Read the model definition and answer for the solid it produces. Units are mm, in the model's axes. Give positions to 0.01 mm unless a question says otherwise; leave off trailing zeros. Order: outer loops, then holes, each group sorted by start corner. A loop starts at its lowest first (then second) coordinate and runs counter-clockwise, first axis right, second up. Notation, with made-up numbers: M -35,89.5 L -13,89.5 A20 cw -13,106.5 Z; hole C 49.5,66 d8. An arc over 180 degrees is marked long. One line per item, written item: value.
from build123d import *

# Parameters (mm, degrees)
SM_START                 = -3
SM_BASE_FLANGE_1_DEPTH   = 6
CUT_EXTRUDE_1_DEPTH      = 231.181450165
CUT_EXTRUDE_1_DEPTH_BACK = 231.181450165
SKETCH_7_W               = 4
SKETCH_7_H               = 47
CHAMFER_2_SIZE           = 8
CHAMFER_2_SIZE_2         = 10.078576046
FILLET_1_R               = 6
CHAMFER_3_SIZE           = 4


with BuildPart() as part:
    # Базовая кромка1: read off the stored shape, not the designer's step
    # Базовая кромка1 outline → Базовая кромка1 (new body)
    with BuildSketch(Plane(origin=(0, 0, 0), x_dir=(0, 0, -1), z_dir=(1, 0, 0)).offset(SM_START)):
        with BuildLine():
            Line((-111.5, 0), (-111.5, 146))
            Line((-111.5, 146), (-153.5, 146))
            Line((-153.5, 146), (-153.5, -71.5))
            ThreePointArc((-153.5, -71.5), (-124.210678119, -142.210678119), (-53.5, -171.5))
            Line((-53.5, -171.5), (53.5, -171.5))
            ThreePointArc((53.5, -171.5), (124.210678119, -142.210678119), (153.5, -71.5))
            Line((153.5, -71.5), (153.5, 146))
            Line((153.5, 146), (111.5, 146))
            Line((111.5, 146), (111.5, 0))
            ThreePointArc((111.5, 0), (0, -111.5), (-111.5, 0))
        make_face()
    extrude(amount=SM_BASE_FLANGE_1_DEPTH)

    # Эскиз7 → Вырез-Вытянуть1 (cut, two sides: drawn at the far end of the back side and taken through both)
    with BuildSketch(Plane(origin=(0, 0, 0), x_dir=(0, 0, -1), z_dir=(1, 0, 0)).offset(-CUT_EXTRUDE_1_DEPTH_BACK)):
        Polygon((72.938816537, -84.333736086), (36.565749578, -105.333736086), (57.565749578, -141.706803045), (93.938816537, -120.706803045), align=None)
        Polygon((-72.938816537, -84.333736086), (-93.938816537, -120.706803045), (-57.565749578, -141.706803045), (-36.565749578, -105.333736086), align=None)
        with Locations((-113.5, 122.5)):
            Rectangle(SKETCH_7_W, SKETCH_7_H)
        with Locations((113.5, 122.5)):
            Rectangle(SKETCH_7_W, SKETCH_7_H)
    extrude(amount=CUT_EXTRUDE_1_DEPTH + CUT_EXTRUDE_1_DEPTH_BACK, mode=Mode.SUBTRACT)

    # Фаска2
    # the kernel refuses this chamfer: 10.078576046, 8 mm, written as the material it takes off along each edge
    with BuildSketch(Plane(origin=(23.573463904, 146, -115.5), x_dir=(0, -1, 0), z_dir=(-1, 0, 0))) as chamfer_2_piece_1:
        Polygon((CHAMFER_2_SIZE, 0), (0, -CHAMFER_2_SIZE), (0, 0), align=None)
    extrude(amount=47.146927807, mode=Mode.SUBTRACT)
    with BuildSketch(Plane(origin=(-23.573463904, 146, 115.5), x_dir=(0, 0, 1), z_dir=(1, 0, 0))) as chamfer_2_piece_2:
        Polygon((CHAMFER_2_SIZE, 0), (0, CHAMFER_2_SIZE), (0, 0), align=None)
    extrude(amount=47.146927807, mode=Mode.SUBTRACT)
    with BuildSketch(Plane(origin=(31.048807118, -84.333736086, -72.938816537), x_dir=(0, -0.8660254037844384, -0.5000000000000006), z_dir=(-1, 0, 0)), Plane(origin=(31.048807118, -105.333736086, 36.565749578), x_dir=(0, -0.8660254037844385, 0.5000000000000004), z_dir=(-1, 0, 0))) as chamfer_2_piece_3:
        with BuildLine():
            Line((CHAMFER_2_SIZE, 0), (-2.56612789, -10.56612789))
            ThreePointArc((-2.56612789, -10.56612789), (-1.195031672, -5.481970258), (0, 0))
            Line((0, 0), (CHAMFER_2_SIZE, 0))
        make_face()
    extrude(amount=62.097614236, mode=Mode.SUBTRACT)
    with BuildSketch(Plane(origin=(-29.036718462, -105.333736086, -36.565749578), x_dir=(0, -0.2924871420802376, 0.9562694556022036), z_dir=(1, 0, 0))) as chamfer_2_piece_4:
        with BuildLine():
            Line((8.31589202, 0), (-CHAMFER_2_SIZE_2 * 0.224833432478, CHAMFER_2_SIZE_2 * 0.974397212447))
            Line((-CHAMFER_2_SIZE_2 * 0.224833432478, CHAMFER_2_SIZE_2 * 0.974397212447), (0, 0))
            ThreePointArc((0, 0), (4.305979523, 0.077455676), (8.31589202, 0))
        make_face()
    extrude(amount=58.073436924, mode=Mode.SUBTRACT)
    with BuildSketch(Plane(origin=(29.036718462, -84.333736086, 72.938816537), x_dir=(0, 0.6819100703745066, 0.7314360231228946), z_dir=(-1, 0, 0))) as chamfer_2_piece_5:
        with BuildLine():
            Line((8.31589202, 0), (-CHAMFER_2_SIZE_2 * 0.224833432478, -CHAMFER_2_SIZE_2 * 0.974397212447))
            Line((-CHAMFER_2_SIZE_2 * 0.224833432478, -CHAMFER_2_SIZE_2 * 0.974397212447), (0, 0))
            ThreePointArc((0, 0), (4.305979523, -0.077455676), (8.31589202, 0))
        make_face()
    extrude(amount=58.073436924, mode=Mode.SUBTRACT)

    # Скругление1
    fillet_1_edges = [part.edges().sort_by_distance(p)[0] for p in [
        (0, -120.706803045, -93.938816537),
        (0, -141.706803045, -57.565749578),
        (0, -141.706803045, 57.565749578),
        (0, -120.706803045, 93.938816537),
    ]]
    fillet(fillet_1_edges, radius=FILLET_1_R)

    # Фаска3
    chamfer_3_edges = [part.edges().sort_by_distance(p)[0] for p in [
        (0, 99, -111.5),
        (0, 99, 111.5),
    ]]
    chamfer(chamfer_3_edges, length=CHAMFER_3_SIZE - 0.0001)  # a hair under: the kernel refuses the full size


solid = part.part
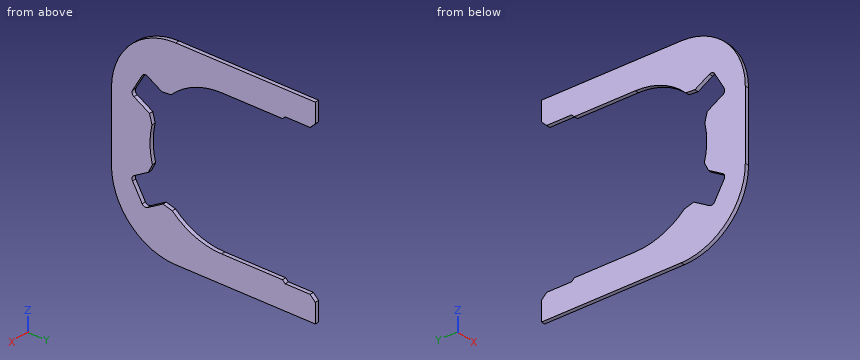
1) Find section A-A, the plane y = 103.5. Write down the section's boundary in (x, z).
Reported:
outline: M -3,-153.5 L 3,-153.5 L 3,-115.5 L -3,-115.5 Z; M -3,115.5 L 3,115.5 L 3,153.5 L -3,153.5 Z
2) Consider probe 1 along Z at (x, y) = (0.5, 101.5); probe 2 along Z at (x, y) = (2.25, 46); probe 3 along Z at (x, y) = (-2, -130). Determine where each line is inside the solid, lowest interval first.
Reported:
probe 1: z = -153.5 to -115.5, 115.5 to 153.5
probe 2: z = -153.5 to -111.5, 111.5 to 153.5
probe 3: z = -134.6 to -77.84, -50.81 to 50.81, 77.84 to 134.6
3) Find section C-C, the plane y = 21. Write down the section's boundary in (x, z), plus the area to 3 significant figures.
Reported:
outline: M -3,-153.5 L 3,-153.5 L 3,-111.5 L -3,-111.5 Z; M -3,111.5 L 3,111.5 L 3,153.5 L -3,153.5 Z
area: 504 mm^2
4) This flat-tipped pin is pushed along its axis until it touches: pin 1 Ø2 at (x, z) = (-0.5, -118.5) entering from +Y. Where does it stop, or does it pass through?
Reported:
pin 1: stops at y = 142
5) Find section D-D, the plane z = -19.5. Write down the section's boundary in (x, y), plus the area to 3 significant figures.
Reported:
outline: M -3,-171.5 L 3,-171.5 L 3,-109.78 L -3,-109.78 Z
area: 370 mm^2
